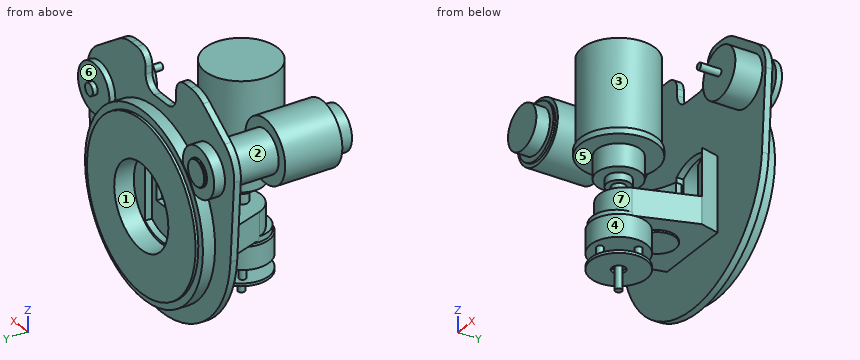
from build123d import *

# Parameters (mm, degrees)
ESTRUSIONE_ESTRUSIONE1_DEPTH      = 40
ESTRUSIONE_ESTRUSIONE2_DEPTH      = 70
SCHIZZO27_W                       = 50.85998704
SCHIZZO27_H                       = 8.16
ESTRUSIONE_ESTRUSIONE10_DEPTH     = 22.131
ESTRUSIONE_ESTRUSIONE5_DEPTH      = 3
ESTRUSIONE_ESTRUSIONE5_DEPTH_BACK = 5
SCHIZZO9_W                        = 33
SCHIZZO9_H                        = 41.5
SCHIZZO14_R                       = 5
ESTRUSIONE_ESTRUSIONE6_DEPTH      = 19
SCHIZZO15_R                       = 41.5
SCHIZZO15_R_2                     = 10
ESTRUSIONE_ESTRUSIONE7_DEPTH      = 4
SCHIZZO16_R                       = 5
ESTRUSIONE_ESTRUSIONE8_DEPTH      = 53
ESTRUSIONE_ESTRUSIONE9_DEPTH      = 10


# Read off the part's stored shape, not the designer's step: Estrusione-Estrusione2
with BuildPart() as part:
    # Schizzo1 → Estrusione-Estrusione1 (new body)
    with BuildSketch(Plane.XY):
        with BuildLine():
            Line((-35.838179279, -60.454520749), (-64.807485396, 23.440548807))
            ThreePointArc((-64.807485396, 23.440548807), (-64.915106011, 24.005921967), (-64.857270382, 24.57853357))
            Line((-64.857270382, 24.57853357), (-57.99999352, 52))
            Line((-57.99999352, 52), (57.99999352, 52))
            Line((57.99999352, 52), (64.857270382, 24.57853357))
            ThreePointArc((64.857270382, 24.57853357), (64.915106011, 24.005921967), (64.807485396, 23.440548807))
            Line((64.807485396, 23.440548807), (35.838179279, -60.454520749))
            ThreePointArc((35.838179279, -60.454520749), (0, -85.994059495), (-35.838179279, -60.454520749))
        make_face()
    extrude(amount=ESTRUSIONE_ESTRUSIONE1_DEPTH)

    # Estrusione-Estrusione2 outline → Estrusione-Estrusione2 (add)
    with BuildSketch(Plane.XY.offset(40)):
        with BuildLine():
            Line((57.99999352, 52), (25.42999352, 52))
            Line((25.42999352, 52), (25.42999352, 43.84))
            ThreePointArc((25.42999352, 43.84), (46.220051809, 36.161219578), (64.910772431, 24.251259249))
            ThreePointArc((64.910772431, 24.251259249), (64.890816245, 24.416007214), (64.857270382, 24.57853357))
            Line((64.857270382, 24.57853357), (57.99999352, 52))
        make_face()
        with BuildLine():
            Line((-25.42999352, 52), (-57.99999352, 52))
            Line((-57.99999352, 52), (-64.857270382, 24.57853357))
            ThreePointArc((-64.857270382, 24.57853357), (-64.890816245, 24.416007214), (-64.910772431, 24.251259249))
            ThreePointArc((-64.910772431, 24.251259249), (-46.220051809, 36.161219578), (-25.42999352, 43.84))
            Line((-25.42999352, 43.84), (-25.42999352, 52))
        make_face()
    extrude(amount=ESTRUSIONE_ESTRUSIONE2_DEPTH)

    # Schizzo27 → Estrusione-Estrusione10 (add)
    with BuildSketch(Plane.XY.offset(40)):
        with Locations((0, 47.92)):
            Rectangle(SCHIZZO27_W, SCHIZZO27_H)
    extrude(amount=ESTRUSIONE_ESTRUSIONE10_DEPTH)

    # Schizzo12 → Estrusione-Estrusione5 (add, two sides: drawn at the far end of the back side and taken through both)
    with BuildSketch(Plane(origin=(0, 0, 0), x_dir=(-1, 0, 0), z_dir=(0, 0, -1)).offset(-ESTRUSIONE_ESTRUSIONE5_DEPTH_BACK)):
        with BuildLine():
            ThreePointArc((8.764790291, -25.537784774), (0, 27), (-8.764790291, -25.537784774))
            ThreePointArc((-8.764790291, -25.537784774), (0, -96.454520749), (8.764790291, -25.537784774))
        make_face()
    extrude(amount=ESTRUSIONE_ESTRUSIONE5_DEPTH + ESTRUSIONE_ESTRUSIONE5_DEPTH_BACK)

    # Schizzo9 → Rivoluzione4 (revolve)
    with BuildSketch(Plane(origin=(0, 0, 0), x_dir=(0, 0, -1), z_dir=(1, 0, 0))):
        Polygon((-40, -46.994520749), (-59.49, -46.994520749), (-59.49, -39.494520749), (-70.49, -39.494520749), (-70.49, -24.494520749), (-103.49, -24.494520749), (-103.49, -0.244520749), (-112.49, -0.244520749), (-112.49, -2.994520749), (-242.49, -2.994520749), (-242.49, -56.994520749), (-40, -56.994520749), align=None)
        with Locations((19.5, -36.244520749)):
            Rectangle(SCHIZZO9_W, SCHIZZO9_H)
    revolve(axis=Axis((0, -56.994520749, 40), (0, 0, 1)))

    # Schizzo14 → Estrusione-Estrusione6 (add)
    with BuildSketch(Plane(origin=(0, 0, -36), x_dir=(-1, 0, 0), z_dir=(0, 0, -1))):
        with Locations((0, -84.661187416)):
            Circle(SCHIZZO14_R)
        with Locations((-23.962922923, -43.156187416)):
            Circle(SCHIZZO14_R)
        with Locations((23.962922923, -43.156187416)):
            Circle(SCHIZZO14_R)
    extrude(amount=ESTRUSIONE_ESTRUSIONE6_DEPTH)

    # Schizzo15 → Estrusione-Estrusione7 (add)
    with BuildSketch(Plane(origin=(0, 0, -55), x_dir=(-1, 0, 0), z_dir=(0, 0, -1))):
        with Locations(Location((0, -56.994520749, 0), (0, 0, 90))):
            Circle(SCHIZZO15_R)
        with Locations(Location((0, -56.994520749, 0), (0, 0, 90))):
            Circle(SCHIZZO15_R_2, mode=Mode.SUBTRACT)
    extrude(amount=ESTRUSIONE_ESTRUSIONE7_DEPTH)

    # Schizzo16 → Estrusione-Estrusione8 (add)
    with BuildSketch(Plane(origin=(0, 0, -36), x_dir=(-1, 0, 0), z_dir=(0, 0, -1))):
        with Locations((0, -56.994520749)):
            Circle(SCHIZZO16_R)
    extrude(amount=ESTRUSIONE_ESTRUSIONE8_DEPTH)

    # Schizzo17 → Estrusione-Estrusione9 (add)
    with BuildSketch(Plane(origin=(0, 52, 0), x_dir=(1, 0, 0), z_dir=(0, 1, 0))):
        with BuildLine():
            Line((-159.445, -66.608848829), (-167.720236988, -184.359565795))
            ThreePointArc((-167.720236988, -184.359565795), (-162.859060274, -209.626630738), (-146.076696991, -229.130678845))
            Line((-146.076696991, -229.130678845), (-96.455754418, -263.080519362))
            ThreePointArc((-96.455754418, -263.080519362), (-82.999085751, -269.581228991), (-68.222312421, -271.814640564))
            Line((-68.222312421, -271.814640564), (-54.96, -271.814640564))
            ThreePointArc((-54.96, -271.814640564), (-40.817864376, -265.956776188), (-34.96, -251.814640564))
            Line((-34.96, -251.814640564), (-34.96, -241.814640564))
            ThreePointArc((-34.96, -241.814640564), (-29.102135624, -227.67250494), (-14.96, -221.814640564))
            Line((-14.96, -221.814640564), (14.96, -221.814640564))
            ThreePointArc((14.96, -221.814640564), (29.102135624, -227.67250494), (34.96, -241.814640564))
            Line((34.96, -241.814640564), (34.96, -251.814640564))
            ThreePointArc((34.96, -251.814640564), (40.817864376, -265.956776188), (54.96, -271.814640564))
            Line((54.96, -271.814640564), (68.222312421, -271.814640564))
            ThreePointArc((68.222312421, -271.814640564), (82.999085751, -269.581228991), (96.455754418, -263.080519362))
            Line((96.455754418, -263.080519362), (146.076696991, -229.130678845))
            ThreePointArc((146.076696991, -229.130678845), (162.859060274, -209.626630738), (167.720236988, -184.359565795))
            Line((167.720236988, -184.359565795), (159.445, -66.608848829))
            ThreePointArc((159.445, -66.608848829), (0, 82.024), (-159.445, -66.608848829))
        make_face()
        with BuildLine():
            Line((-36, -30.9285), (-36, -125.0235))
            ThreePointArc((-36, -125.0235), (0, -136.545782144), (36, -125.0235))
            Line((36, -125.0235), (36, -30.9285))
            ThreePointArc((36, -30.9285), (0, -19.406217856), (-36, -30.9285))
        make_face(mode=Mode.SUBTRACT)
    extrude(amount=ESTRUSIONE_ESTRUSIONE9_DEPTH)

    # Schizzo19 → Rivoluzione5 (revolve)
    with BuildSketch(Plane(origin=(0, 0, 0), x_dir=(0, 0, -1), z_dir=(1, 0, 0))):
        Polygon((57.024, 87), (57.024, 69), (12.024, 69), (12.024, 62), (-15.976, 62), (-15.976, 91), (46.524, 91), (46.524, 87), align=None)
    revolve(axis=Axis((0, -948, 77.976), (0, 1, 0)))

    # Schizzo23 → Rivoluzione6 (revolve)
    with BuildSketch(Plane.XY.offset(185.24165124)):
        Polygon((-123.395016366, 62), (-138.395016366, 62), (-138.395016366, 70.1), (-159.395016366, 70.1), (-159.395016366, 86.1), (-142.895016366, 86.1), (-142.895016366, 88.6), (-141.895016366, 89.6), (-123.395016366, 89.6), align=None)
        Polygon((-123.395016366, 52), (-154.395016366, 52), (-154.395016366, -12.6), (-169.395016366, -12.6), (-169.395016366, -97.1), (-163.895016366, -97.1), (-163.895016366, -100.1), (-155.895016366, -100.1), (-155.895016366, -120.1), (-123.395016366, -120.1), align=None)
    revolve(axis=Axis((-123.395016366, 62, 185.24165124), (0, -1, 0)))

    # Schizzo24 → Rivoluzione7 (revolve)
    with BuildSketch(Plane.XY.offset(185.24165124), mode=Mode.PRIVATE) as rivoluzione7_sk:
        Polygon((123.4, 62), (123.4, 88.7), (132.4, 88.7), (132.4, 81.7), (159.4, 81.7), (159.4, 73), (132.4, 73), (132.4, 62), align=None)
        Polygon((123.4, 52), (123.4, -18), (128.4, -18), (128.4, 12), (160.4, 12), (160.4, 52), align=None)
    revolve(rivoluzione7_sk.sketch.rotate(Axis((123.4, -18, 185.24165124), (0, 1, 0)), 90), axis=Axis((123.4, -18, 185.24165124), (0, 1, 0)))


solid = part.part
Input: part model. Units: mm. Frame: model coordinates. Face numbers are marked on the shaded views. A direction names the side the tool comes from. Coordinates: 2 decimals unless noted, no trailing zeros. Loops run counter-clockwise (first coordinate to the right, second up) from the corner with the lowest first, then second, coordinate; pieces in that order, holes last. Notation, with made-up numbers: (68.5, 45.5) -> (98.5, 45.5) arc R15 cw to (98.5, 70.5) -> close; hole circle Ø6 at (68, -0.5). An arc over 180 degrees is marked (long way). Write item = value, one per line. Start each with the question number.
Item 1: Cut plane C-C, the plane x = 78.5. Return loops of the section in (y, z).
Item 2: Cut plane A-A, the plane x = 0. Count the separate pieces of the cut face and the enclosed holes in it, plus the area to 3 significant figures.
Item 3: First-contact query: P1, Ø1, axis at x = -0.5, y = -7.5, coming from the -Z side; P2, Ø1.5, axis at x = -17, y = -33.5, coming from the +Z side; P3, Ø1.5, axis at x = 113.5, z = 233.5, coming from the -Y side. Flat tips, straight axial feed; report the tip coordinate or a pass-through.
Item 4: Reachability of the marked faces 4, 5, 6 and 7 from +Z, -Z, +X, -X, +Y, -Y: full face, straight path, thin tool, end or side. Return the list, or none.
Item 5: Material intervals for line 1 (Z direction, x = -17, y = -52); line 2 (Y direction, x = 4, z = -40); line 3 (Y direction, x = 90, z = 159), sorted ascending.
Item 6: Mould query, pull axis Z, two halves, no side actions, for the marked faces 1, 2 and 3. Classes: pulls with the +Z half, pulls with the -Z half, needs draft (parallel to the pull), parting line crosses it, or undercut.
Ans:
q1.outline = (52, -61.42) -> (62, -61.42) -> (62, 33.96) -> (69, 33.96) -> (69, -31.85) -> (87, -31.85) -> (87, -18.66) -> (91, -18.66) -> (91, 174.61) -> (87, 174.61) -> (87, 187.81) -> (69, 187.81) -> (69, 122) -> (62, 122) -> (62, 270.75) -> (52, 270.75) -> close
q2.separate_pieces = 3
q2.enclosed_holes = 0
q2.area = 33,200 mm²
q3.P1 = -3
q3.P2 = 242.49
q3.P3 = 52
q4.face_4 = -Z
q4.face_5 = none
q4.face_6 = +Y
q4.face_7 = -Y
q5.line_1 = -59 to -55, -36 to 40, 70.49 to 242.49
q5.line_2 = -87.66 to -81.66, -59.99 to -53.99, 52 to 62, 69 to 91
q5.line_3 = 52 to 62, 69 to 91
q6.face_1 = undercut
q6.face_2 = parting line crosses it
q6.face_3 = needs draft
